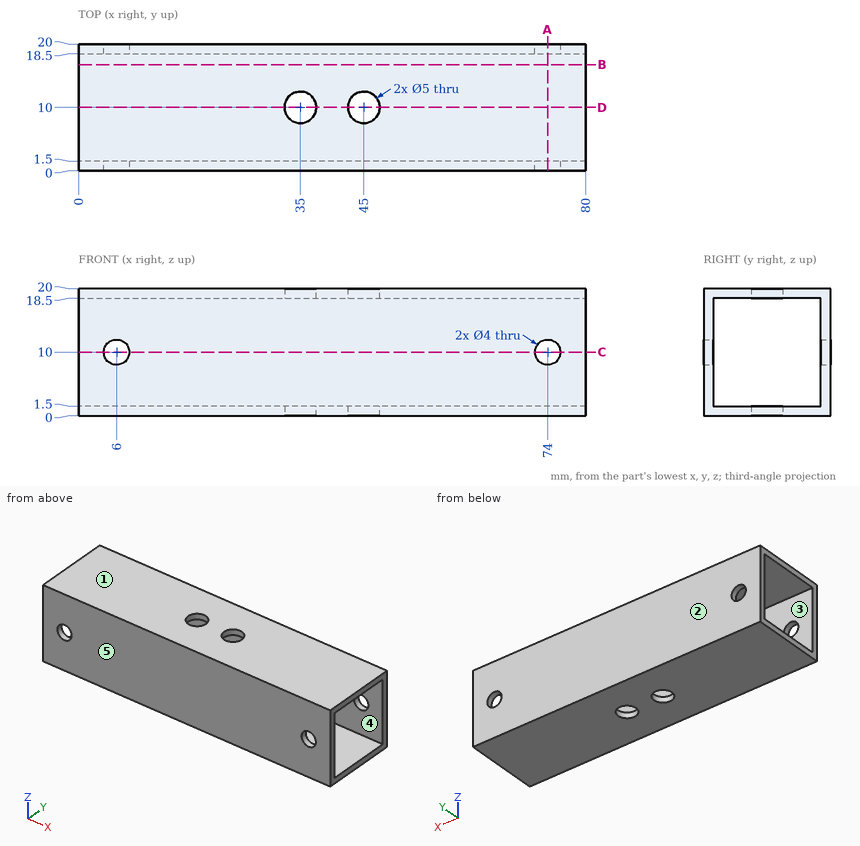
Check sheet for the drawn part. Datum: minimum x, y, z corner. Units: mm. A direction names the side the tool comes from. Give positions to 0.01 mm unless a question says otherwise; leave off trailing zeros. Write each loop counter-clockwise with the first axis right and the second up, starting at its lowest first coordinate (ties: lowest second). Pieces come first, ordered by that corner, then holes. Notation, with made-up numbers: (10.5, -38.75) -> (54.5, -38.75) arc R12 cw to (54.5, -33.75) -> close; hole circle Ø5 at (65.25, 10.25). An arc over 180 degrees is marked (long way). Use one line per item in the form item = value. Start each with the question number.
1. Section check B-B (y = 16.75). Record the cut outline in (x, z), and give its area (3 significant figures).
2. Thickness scan on line 1 along X through (y, z) = (0.65, 10); line 2 along Y through (x, z) = (39, 7.5). Record the ranges inside material, lowest first. Write a range as from..to.
3. Access from +Z, -Z, +X, -X, +Y, -Y to the whole of each face (thin tool, end or side, straight path). Record for the marked faces 4 and 5.
4. Section check C-C (z = 10). Record the cut outline in (x, y), and give its area (3 significant figures).
5. Go/stop test with a flat-tipped pin: P1, Ø5, axis at x = 6, z = 10, coming from the -Y side. Record where the tip stops, or that it passes through.
6. Section check D-D (y = 10). Record the cut outline in (x, z).
7. Section check A-A (x = 74). Record the cut outline in (y, z), and give its area (3 significant figures).
8. Mould release check, pull along Z, two halves, no side actions. Record for the marked faces 1, 2 and 3: pulls with the +Z half, pulls with the -Z half, needs draft (parallel to the pull), parting line crosses it, or undercut.
Conclusion:
q1.outline = (0, 0) -> (80, 0) -> (80, 1.5) -> (0, 1.5) -> close; (0, 18.5) -> (80, 18.5) -> (80, 20) -> (0, 20) -> close
q1.area = 240 mm²
q2.line_1 = 0..4, 8..72, 76..80
q2.line_2 = 0..1.5, 18.5..20
q3.face_4 = +X, -X
q3.face_5 = +Z, -Z, +X, -X, -Y
q4.outline = (0, 0) -> (4, 0) -> (4, 1.5) -> (0, 1.5) -> close; (0, 18.5) -> (4, 18.5) -> (4, 20) -> (0, 20) -> close; (8, 0) -> (72, 0) -> (72, 1.5) -> (8, 1.5) -> close; (8, 18.5) -> (72, 18.5) -> (72, 20) -> (8, 20) -> close; (76, 0) -> (80, 0) -> (80, 1.5) -> (76, 1.5) -> close; (76, 18.5) -> (80, 18.5) -> (80, 20) -> (76, 20) -> close
q4.area = 216 mm²
q5.P1 = 0
q6.outline = (0, 0) -> (32.5, 0) -> (32.5, 1.5) -> (0, 1.5) -> close; (0, 18.5) -> (32.5, 18.5) -> (32.5, 20) -> (0, 20) -> close; (37.5, 0) -> (42.5, 0) -> (42.5, 1.5) -> (37.5, 1.5) -> close; (37.5, 18.5) -> (42.5, 18.5) -> (42.5, 20) -> (37.5, 20) -> close; (47.5, 0) -> (80, 0) -> (80, 1.5) -> (47.5, 1.5) -> close; (47.5, 18.5) -> (80, 18.5) -> (80, 20) -> (47.5, 20) -> close
q7.outline = (0, 0) -> (20, 0) -> (20, 8) -> (18.5, 8) -> (18.5, 1.5) -> (1.5, 1.5) -> (1.5, 8) -> (0, 8) -> close; (0, 12) -> (1.5, 12) -> (1.5, 18.5) -> (18.5, 18.5) -> (18.5, 12) -> (20, 12) -> (20, 20) -> (0, 20) -> close
q7.area = 99.0 mm²
q8.face_1 = pulls with the +Z half
q8.face_2 = needs draft
q8.face_3 = undercut
